```python
from build123d import *

# Parameters (mm, degrees)
BOSS_EXTRUDE1_DEPTH = 110
SHELL1_T            = -2
SKETCH3_W           = 216
SKETCH3_H           = 46
CUT_EXTRUDE1_DEPTH  = 10
BOSS_EXTRUDE2_REACH = 232.002
SKETCH6_R           = 1.5
CUT_EXTRUDE2_DEPTH  = 5


with BuildPart() as part:
    # Sketch2 → Boss-Extrude1 (new, symmetric)
    with BuildSketch(Plane(origin=(0, 0, 0), x_dir=(0, 0, -1), z_dir=(1, 0, 0))):
        Polygon((25, -30), (25, -5.355339059), (-28.033008589, 47.67766953), (-45.710678119, 30), (-45.710678119, -30), (-55.710678119, -30), (-55.710678119, -35), (-45.710678119, -35), (25, -35), (35, -35), (35, -30), align=None)
    extrude(amount=BOSS_EXTRUDE1_DEPTH, both=True)

    # Shell1
    shell1_openings = [part.faces().sort_by_distance(p)[0] for p in [
        (0, 21.161165235, 1.516504294),
    ]]
    offset(amount=SHELL1_T, openings=shell1_openings, kind=Kind.INTERSECTION)

    # Sketch3 → Cut-Extrude1 (cut)
    with BuildSketch(Plane(origin=(0, -33, 0), x_dir=(1, 0, 0), z_dir=(0, 1, 0))):
        Rectangle(SKETCH3_W, SKETCH3_H)
    extrude(amount=-CUT_EXTRUDE1_DEPTH, mode=Mode.SUBTRACT)

    # Sketch5 → Boss-Extrude2 (add, up to next)
    with BuildSketch(Plane(origin=(-108, 0, 0), x_dir=(0, 0, -1), z_dir=(1, 0, 0)), mode=Mode.PRIVATE) as boss_extrude2_sk1:
        Polygon((-36.441125497, 36.441125497), (23, -23), (23, -4.898066402), (17.484567107, -10.413499295), (-32.905591591, 39.976659403), align=None)
    boss_extrude2_tool1 = extrude(boss_extrude2_sk1.sketch, amount=BOSS_EXTRUDE2_REACH, mode=Mode.PRIVATE) - part.part
    add(boss_extrude2_tool1.solids().sort_by_distance((-108, 7.973571, 3.970996))[0])

    # Sketch6 → Cut-Extrude2 (cut, symmetric)
    with BuildSketch(Plane(origin=(0, 3.535533906, -3.535533906), x_dir=(1, 0, 0), z_dir=(0, 0.7071067811865476, -0.7071067811865475))):
        Polygon((-98, 13.636038969), (-108, 13.636038969), (-108, -46.535533906), (-98, -46.535533906), (-98, -51.535533906), (-5, -51.535533906), (-5, -46.535533906), (5, -46.535533906), (5, -51.535533906), (98, -51.535533906), (98, -46.535533906), (108, -46.535533906), (108, 13.636038969), (98, 13.636038969), (98, 18.636038969), (5, 18.636038969), (5, 13.636038969), (-5, 13.636038969), (-5, 18.636038969), (-98, 18.636038969), align=None)
        with Locations(Location((0, 16.136038969, 0), (0, 0, 90))):
            Circle(SKETCH6_R)
        with Locations(Location((-102.5, 16.136038969, 0), (0, 0, 90))):
            Circle(SKETCH6_R)
        with Locations(Location((102.5, 16.136038969, 0), (0, 0, 90))):
            Circle(SKETCH6_R)
        with Locations(Location((102.5, -49.035533906, 0), (0, 0, 90))):
            Circle(SKETCH6_R)
        with Locations(Location((0, -49.035533906, 0), (0, 0, 90))):
            Circle(SKETCH6_R)
        with Locations(Location((-102.5, -49.035533906, 0), (0, 0, 90))):
            Circle(SKETCH6_R)
    extrude(amount=CUT_EXTRUDE2_DEPTH, both=True, mode=Mode.SUBTRACT)


solid = part.part
```
Verification items for the finished model (mm, model axes). A direction names the side the tool comes from. Give positions to 0.01 mm unless a question says otherwise; leave off trailing zeros. Loops run counter-clockwise (first coordinate to the right, second up) from the corner with the lowest first, then second, coordinate; pieces in that order, holes last.
1. Mould release check, pull along Z, two halves, no side actions. Record for faces 6 (the flat face through (0.513, -4.497, -24.142)), 7 (the flat face through (2, -33, -28)), 8 (the flat face through (1.54, 38.96, 36.75)): released by +Z, released by -Z, zero draft, split by the parting line, or undercut.
2. Section check A-A, the plane y = -18.5. Enter the section's corners in (x, z).
3. Section check D-D, the plane z = 40. Enter the section's corners in (x, y), then the cut area to 3 significant figures.
4. Section check C-C, the plane y = 25. Enter the section's corners in (x, z), then the cut area to 3 significant figures.
5. Set-up check for faces 1 (the flat face through (-2, -18, -18)), 2 (the flat face through (98, -10, -13)), 3 (the flat face through (-5, 36, 33)), 4 (the flat face through (2, -33, 39)), 5 (the flat face through (2, -30, 51)): record each of +Z, -Z, +X, -X, +Y, -Y from which the full face is reachable in a straight line by a thin tool's end or side.
6. Go/stop test with flat-tipped pins: pin 1 Ø9 at (x, z) = (-8.5, 42) entering from +Y; pin 2 Ø5 at (x, y) = (25.5, 38.5) entering from +Z; pin 3 Ø10 at (x, z) = (62.5, -16.5) entering from +Y. Record where each tip stops, or that it passes through.
7. Section check B-B, the plane x = -70. Enter the section's corners in (y, z), then the cut area to 3 significant figures.
8. Thickness scan on line 1 (X direction, y = 18.5, z = 34); line 2 (Z direction, x = -59, y = -29); line 3 (Z direction, x = -60, y = 3.5). Record the ranges inside material, lowest first.
Geometry says:
1. face 6: released by -Z
1. face 7: undercut
1. face 8: released by +Z
2. outline: (-110, -25) - (110, -25) - (110, 45.71) - (-110, 45.71) - close; hole (-108, -18.5) - (108, -18.5) - (108, 43.71) - (-108, 43.71) - close
3. outline: (-110, -35) - (110, -35) - (110, 35.71) - (-110, 35.71) - close; hole (-108, -33) - (108, -33) - (108, 32.88) - (-108, 32.88) - close
3. area: 1,330 mm2
4. outline: (-110, 5.36) - (-108, 5.36) - (-108, 43.71) - (108, 43.71) - (108, 5.36) - (110, 5.36) - (110, 45.71) - (-110, 45.71) - close
4. area: 593 mm2
5. face 1: -Y
5. face 2: +Y
5. face 3: -Z
5. face 4: none
5. face 5: +Z, +X, -X, +Y
6. pin 1: stops at y = 38.21
6. pin 2: stops at z = 39.71
6. pin 3: stops at y = -6.4
7. outline: (-35, -35) - (-30, -35) - (-30, -25) - (-5.36, -25) - (-3.36, -23) - (-4.9, -23) - (-10.41, -17.48) - (-9.64, -16.71) - (-13.18, -13.18) - (-23, -23) - (-32, -23) - (-32, -33) - (-33, -33) - (-33, -23) - (-35, -23) - close; (-35, 23) - (-33, 23) - (-33, 53.71) - (-32, 53.71) - (-32, 43.71) - (29.17, 43.71) - (46.26, 26.62) - (47.68, 28.03) - (30, 45.71) - (-30, 45.71) - (-30, 55.71) - (-35, 55.71) - close
7. area: 448 mm2
8. line 1: x = -110 to -108, 108 to 110
8. line 2: z = -25 to -23, 43.71 to 45.71
8. line 3: z = 43.71 to 45.71
